Can you work these out from the model? Positions are in its coordinate system, mm. Face numbers are marked on the shaded views. A direction names the side the tool comes from. Round coordinates to 2 decimals unless told otherwise and drop trailing zeros. Loops run counter-clockwise (first coordinate to the right, second up) from the corner with the lowest first, then second, coordinate; pieces in that order, holes last.
(1) I want a section at A-A on x = 70. Write out the boundary of the cut face in (y, z).
(2) Will these pins go through, and if not, where does the flat tip stop? pin 1 Ø5 at (x, y) = (55, -1.5) entering from -Z; pin 2 Ø6 at (x, z) = (20, 5) entering from -Y; pin 3 Ø6 at (y, z) = (6.5, 8) entering from +X.
(3) I want a section at B-B on y = 3. Write out the boundary of the cut face in (x, z).
(4) If I drill on line 1 along Y through (x, z) = (25.5, 10.5); line 2 along Y through (x, z) = (31, 6.25); line 3 along X through (y, z) = (-1, 9.75) (3 decimals), over which ranges is the centre line in solid material (lowest first)?
(5) Which directions (+Z, -Z, +X, -X, +Y, -Y) give clear straight access to the entire face, cutting with the end or side of a thin tool? Please do the marked faces 1 and 2.
from build123d import *

# Parameters (mm, degrees)
F0_W         = 30
F0_H         = 12
F1_DEPTH     = 16
F3_DEPTH     = 200
F5_DEPTH     = 30
F7_DEPTH     = 10
F8_T4_DEPTH  = 52
F8_S5_R      = 6
F8_T6_DEPTH  = 28
F8_T10_DEPTH = 52
F8_S11_R     = 6
F8_T12_DEPTH = 28
F9_SIZE      = 1.99999


# Not quite as in the source:
# - a fillet or chamfer that OpenCascade refuses, or shapes differently, is made with other operations: its cross-section is extruded or revolved along the edge and cut away or added
# - a fillet or chamfer is up to 0.001 mm smaller than in the source, because OpenCascade refuses the exact size


with BuildPart() as f1:
    # F0 (on Front) → F1 (new body)
    with BuildSketch(Plane.XZ):
        with Locations((15, 6)):
            Rectangle(F0_W, F0_H)
    extrude(amount=F1_DEPTH)

    # F2 (on face) → F3 (join)
    with BuildSketch(Plane.YZ.offset(30)):
        with BuildLine():
            ThreePointArc((-8, 0), (-3.7573593129, 1.7573593129), (-2, 6))
            ThreePointArc((-2, 6), (-3.7573593129, 10.2426406871), (-8, 12))
            ThreePointArc((-8, 12), (-14, 6), (-8, 0))
        make_face()
    extrude(amount=F3_DEPTH)

    # F4 (on face) → F5 (join)
    with BuildSketch(Plane.YZ.offset(230)):
        with BuildLine():
            Line((-8, 12), (-16, 12))
            Line((-16, 12), (-16, 0))
            Line((-16, 0), (-8, 0))
            ThreePointArc((-8, 0), (-14, 6), (-8, 12))
        make_face()
        with BuildLine():
            Line((0, 12), (-8, 12))
            ThreePointArc((-8, 12), (-3.7573593129, 10.2426406871), (-2, 6))
            ThreePointArc((-2, 6), (-3.7573593129, 1.7573593129), (-8, 0))
            Line((-8, 0), (0, 0))
            Line((0, 0), (0, 12))
        make_face()
        with BuildLine():
            ThreePointArc((-2, 6), (-3.7573593129, 10.2426406871), (-8, 12))
            ThreePointArc((-8, 12), (-14, 6), (-8, 0))
            ThreePointArc((-8, 0), (-3.7573593129, 1.7573593129), (-2, 6))
        make_face()
    extrude(amount=F5_DEPTH)

    # F6 (on face) → F7 (join)
    with BuildSketch(Plane.XY.offset(12)):
        with BuildLine():
            ThreePointArc((241.6696972202, -16), (264.0861928738, -27.5781262586), (280, -8))
            ThreePointArc((280, -8), (264.0861928738, 11.5781262586), (241.6696972202, 0))
            Line((241.6696972202, 0), (260, 0))
            Line((260, 0), (260, -16))
            Line((260, -16), (241.6696972202, -16))
        make_face()
    extrude(amount=-F7_DEPTH)

    # F8: fillet of radius 8 on 2 edges, made by hand


with BuildPart() as f8_tool2:
    # F8_s3 → F8_t4 (new body)
    with BuildSketch(Plane.XY.offset(-20)):
        with BuildLine():
            ThreePointArc((230, -8), (232.3431457505, -2.3431457505), (238, 0))
            Line((238, 0), (230, 0))
            Line((230, 0), (230, -8))
        make_face()
    extrude(amount=F8_T4_DEPTH)

    # F8_s5 → F8_t6 (cut, symmetric)
    with BuildSketch(Plane.YZ.offset(234)):
        with Locations((-8, 6)):
            Circle(F8_S5_R)
    extrude(amount=F8_T6_DEPTH, both=True, mode=Mode.SUBTRACT)


with BuildPart() as f1_1:
    add(f1.part)

    # F8_t1: cut F8_tool2
    add(f8_tool2.part, mode=Mode.SUBTRACT)


with BuildPart() as f8_tool8:
    # F8_s9 → F8_t10 (new body)
    with BuildSketch(Plane.XY.offset(32)):
        with BuildLine():
            ThreePointArc((230, -8), (232.3431457505, -13.6568542495), (238, -16))
            Line((238, -16), (230, -16))
            Line((230, -16), (230, -8))
        make_face()
    extrude(amount=-F8_T10_DEPTH)

    # F8_s11 → F8_t12 (cut, symmetric)
    with BuildSketch(Plane.YZ.offset(234)):
        with Locations((-8, 6)):
            Circle(F8_S11_R)
    extrude(amount=F8_T12_DEPTH, both=True, mode=Mode.SUBTRACT)


with BuildPart() as f1_2:
    add(f1_1.part)

    # F8_t7: cut F8_tool8
    add(f8_tool8.part, mode=Mode.SUBTRACT)

    # F9 (size 2 in the source; OpenCascade refuses exactly that, so slightly less here)
    f9_edges = [f1_2.edges().sort_by_distance(p)[0] for p in [
        (260, -8, 0),
    ]]
    chamfer(f9_edges, length=F9_SIZE)


solid = f1_2.part
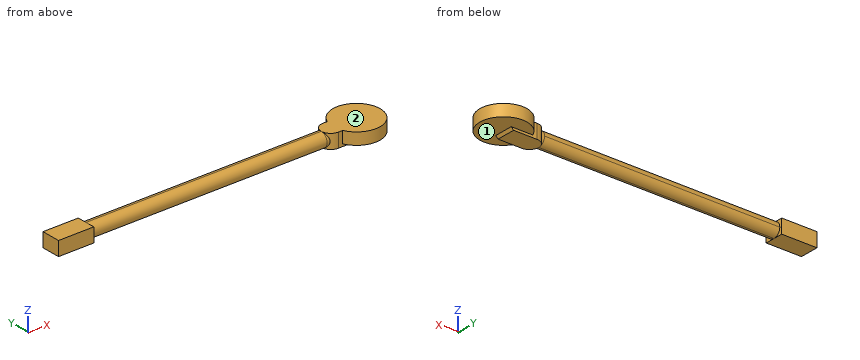
Filled sheet:
1. outline: circle Ø12 at (-8, 6)
2. pin 1: stops at z = 1.53
2. pin 2: stops at y = -16
2. pin 3: stops at x = 276.36
3. outline: (243.3, 2) - (276.7, 2) - (276.7, 12) - (243.3, 12) - close
4. line 1: y = -16 to 0
4. line 2: y = -13.99 to -2.01
4. line 3: x = 0 to 30, 234.127 to 278.735
5. face 1: -Z, +X
5. face 2: +Z, +X, -X, +Y, -Y
